from build123d import *

# Parameters (mm, degrees)
SKETCH1_W           = 150
SKETCH1_H           = 150
SKETCH1_R           = 1.5
BOSS_EXTRUDE1_DEPTH = 5


with BuildPart() as part:
    # Sketch1 → Boss-Extrude1 (new body)
    with BuildSketch(Plane(origin=(0, 0, 0), x_dir=(1, 0, 0), z_dir=(0, 1, 0))):
        with Locations((75, 75)):
            Rectangle(SKETCH1_W, SKETCH1_H)
        with Locations((10, 125)):
            Circle(SKETCH1_R, mode=Mode.SUBTRACT)
        with Locations((10, 100)):
            Circle(SKETCH1_R, mode=Mode.SUBTRACT)
        with BuildLine():
            Line((25, 79.25), (125, 79.25))
            ThreePointArc((125, 79.25), (129.25, 75), (125, 70.75))
            Line((125, 70.75), (25, 70.75))
            ThreePointArc((25, 70.75), (20.75, 75), (25, 79.25))
        make_face(mode=Mode.SUBTRACT)
    extrude(amount=BOSS_EXTRUDE1_DEPTH)


solid = part.part
Geometry: final body of the model. Coordinates: model frame, mm. A direction names the side the tool comes from. Give positions to 0.01 mm unless a question says otherwise; leave off trailing zeros. Write each loop counter-clockwise with the first axis right and the second up, starting at its lowest first coordinate (ties: lowest second). Pieces come first, ordered by that corner, then holes. Notation, with made-up numbers: (49, -37.75) - (78, -37.75) arc R23 ccw to (78, -9.75) - close; hole circle Ø1 at (7.5, 34). An arc over 180 degrees is marked (long way). Return JSON: item names as keys, results as strings. Group by question number.
1) Line query: line 1 (Z direction, x = 10, y = 3.4); line 2 (Z direction, x = 39.5, y = 0.4); line 3 (X direction, y = 3.6, z = -100). Output: solid intervals per line, ascending.
2) First-contact query: P1, Ø2.5, axis at x = 10, z = -100, coming from the +Y side. Flat tip, straight axial feed; report the tip coordinate or a pass-through.
3) Mould query, pull axis X, two halves, no side actions, for faces 3 (the flat face through (76, 2, -70.75)), 4 (the flat face through (0, 2, -74)), 5 (the flat face through (74, 5, -59)). Classes: released by +X, released by -X, zero draft, split by the parting line, or undercut.
4) Set-up query: faces 1 (the flat face through (74, 2, -79.25)), 2 (the flat face through (150, 2, -74)). Return all of +Z, -Z, +X, -X, +Y, -Y with unobstructed straight access to the full face (end or side cutting, diameter ignored); none if empty.
5) Section C-C on z = -75. Return the cut outline in (x, y).
6) Section A-A on x = 106.5. Return the cut outline in (y, z).
7) Section B-B on y = 3.1. Return the cut outline in (x, z), plus the area to 3 significant figures.
Filled in:
{
 "1": {"line 1": "z = -150 to -126.5, -123.5 to -101.5, -98.5 to 0", "line 2": "z = -150 to -79.25, -70.75 to 0", "line 3": "x = 0 to 8.5, 11.5 to 150"},
 "2": {"P1": "passes through"},
 "3": {"face 3": "undercut", "face 4": "released by -X", "face 5": "zero draft"},
 "4": {"face 1": "+Y, -Y", "face 2": "+Z, -Z, +X, +Y, -Y"},
 "5": {"outline": "(0, 0) - (20.75, 0) - (20.75, 5) - (0, 5) - close; (129.25, 0) - (150, 0) - (150, 5) - (129.25, 5) - close"},
 "6": {"outline": "(0, -150) - (5, -150) - (5, -79.25) - (0, -79.25) - close; (0, -70.75) - (5, -70.75) - (5, 0) - (0, 0) - close"},
 "7": {"outline": "(0, -150) - (150, -150) - (150, 0) - (0, 0) - close; hole circle Ø3 at (10, -125); hole circle Ø3 at (10, -100); hole (25, -79.25) - (125, -79.25) arc R4.25 ccw to (125, -70.75) - (25, -70.75) arc R4.25 ccw to start", "area": "21,600 mm^2"}
}
